Autodesk Inventor part; units mm, degrees
ref_plane "YZ Plane" through (0, 0, 0) normal (1, 0, 0) x (0, 1, 0)
ref_plane "XZ Plane" through (0, 0, 0) normal (0, 1, 0) x (-1, 0, 0)
ref_plane "XY Plane" through (0, 0, 0) normal (0, 0, 1) x (1, 0, 0)
sketch "Sketch1" plane through (0, 0, 0) normal (0, 0, 1) x (1, 0, 0)
  circle A0 centre (0, 0) radius 1.75
  circle A1 centre (0, 0) radius 3.75
  dimension "d0" = 3.5
  dimension "d1" = 2
extrude "Extrusion1" add sketch "Sketch1" along normal blind 2
fillet "Fillet1" radius 0.5 1 edges at (-3.75, 0, 0)
sketch "Sketch2" plane through (0, 0, 2) normal (0, 0, 1) x (1, 0, 0)
  circle A0 centre (0, 0) radius 3.75
extrude "Extrusion2" add sketch "Sketch2" along normal blind 1
properties part number "direksiyon mili tutucu"
Source: CAD feature listing. Evaluate the final solid. Frame: model axes, mm. A direction names the side the tool comes from. Round coordinates to 2 decimals unless told otherwise and drop trailing zeros. Loops run counter-clockwise (first coordinate to the right, second up) from the corner with the lowest first, then second, coordinate; pieces in that order, holes last. Notation, with made-up numbers: (-21.5, 87.5) - (12.5, 87.5) arc R21 ccw to (12.5, 101.5) - close; hole circle Ø5 at (48, 14.5). An arc over 180 degrees is marked (long way). Use CSV: the item, a comma, the result in double quotes.
Q1. Section query A-A, the plane x = 0. Output: boundary loops of the cut face in (y, z).
Reported:
outline,"(-3.75, 0.5) arc R0.5 ccw to (-3.25, 0) - (-1.75, 0) - (-1.75, 2) - (1.75, 2) - (1.75, 0) - (3.25, 0) arc R0.5 ccw to (3.75, 0.5) - (3.75, 3) - (-3.75, 3) - close"
Q2. Section query C-C, the plane z = 1.4. Output: boundary loops of the cut face in (x, y).
Reported:
outline,"circle Ø7.5 at (0, 0); hole circle Ø3.5 at (0, 0)"
Q3. Section query D-D, the plane z = 2.3. Output: boundary loops of the cut face in (x, y), then the cut area to 3 significant figures.
Reported:
outline,"circle Ø7.5 at (0, 0)"
area,"44.2 mm^2"
Q4. Reachability of faces 1 (the flat face through (1.4, -1.4, 0)), 2 (the flat face through (0, 0, 2)) from +Z, -Z, +X, -X, +Y, -Y: full face, straight path, thin tool, end or side. Return the list, or none.
Reported:
face 1,"-Z, +X, -X, +Y, -Y"
face 2,"-Z"
Q5. Ray query, line 1 along Y through (x, z) = (0, 0.95); line 2 along Z through (x, y) = (1, 0.5); line 3 along Y through (x, z) = (-0.75, 0.95). Return the intervals inside material, ascending.
Reported:
line 1,"-3.75 to -1.75, 1.75 to 3.75"
line 2,"2 to 3"
line 3,"-3.67 to -1.58, 1.58 to 3.67"
Q6. Mould query, pull axis Y, two halves, no side actions, for faces 3 (the cylindrical face through (-3.746, -0.165, 1.732)), 4 (the cylindrical face through (1.617, 0.67, 0.986)), 5 (the flat face through (0, 0, 3)). Classes: pulls with the +Y half, pulls with the -Y half, needs draft (parallel to the pull), parting line crosses it, or undercut.
Reported:
face 3,"parting line crosses it"
face 4,"undercut"
face 5,"needs draft"
